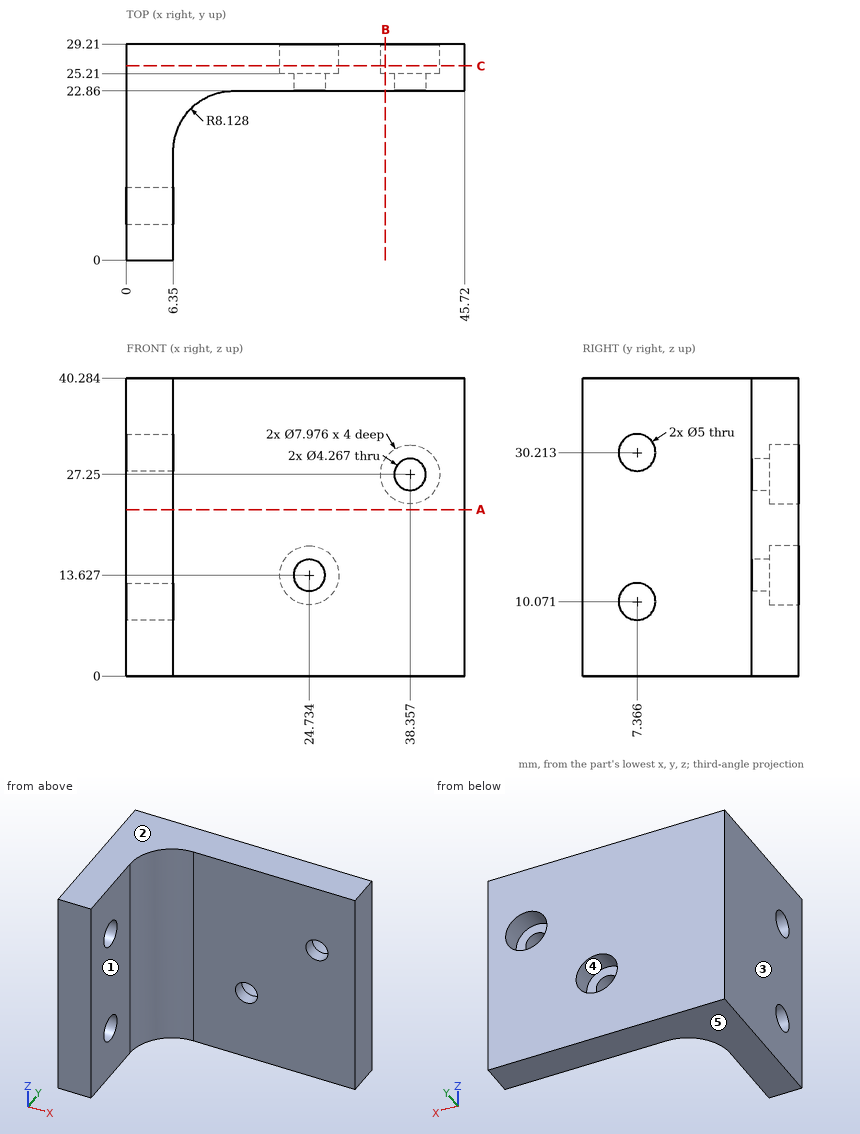
Design review of the part shown in the three views and the two pictorial views. Dimensions are in mm from the part's minimum x, y and z. A direction names the side the tool comes from. Give positions to 0.01 mm unless a question says otherwise; leave off trailing zeros. Write each loop counter-clockwise with the first axis right and the second up, starting at its lowest first coordinate (ties: lowest second). Pieces come first, ordered by that corner, then holes. Notation, with made-up numbers: M 16,15.5 L 32,15.5 A15 cw 32,42.5 Z; hole C -17,-29.75 d3. An arc over 180 degrees is marked long. One line per item, written item: value.
1) For line 1 (Y direction, x = 28, z = 33); line 2 (X direction, y = 11, z = 23.5); line 3 (Z direction, x = 5.5, y = 9.5) (1 decimal), list the stretches that pass through material, from the lowest coordinate up. Write a range as from..to.
Results are:
line 1: y = 22.86..29.21
line 2: x = 0..6.35
line 3: z = 0..8.8, 11.4..28.9, 31.5..40.3
2) Take a section at C-C, the plane y = 26.25. Count the separate pieces of the cut face and the enclosed holes in it, then the cut area to 3 significant figures.
Results are:
separate pieces: 1
enclosed holes: 2
area: 1,740 mm²
3) Take a section at B-B, the plane x = 35. Write out the cut boundary in (y, z) (1 decimal).
Results are:
outline: M 22.9,0 L 29.2,0 L 29.2,25.1 L 25.2,25.1 L 25.2,29.4 L 29.2,29.4 L 29.2,40.3 L 22.9,40.3 Z
4) For the marked faces 1 and 2, list the 3-axis set-ups (+Z, -Z, +X, -X, +Y, -Y) from which the entire face can be reached by the end or side of a thin tool; tool diameter is ignored.
Results are:
face 1: +Z, -Z, +X, -Y
face 2: +Z, +X, -X, +Y, -Y
5) Take a section at A-A, the plane z = 22.5. Write out the cut boundary in (x, y), then the cut area to 3 significant figures.
Results are:
outline: M 0,0 L 6.35,0 L 6.35,14.73 A8.13 cw 14.48,22.86 L 45.72,22.86 L 45.72,29.21 L 0,29.21 Z
area: 450 mm²
6) For P1, Ø5, axis at y = 15, z = 23, coming from the +X side (1 decimal); P2, Ø9, axis at x = 24.5, z = 14.5, coming from the +Y side; P3, Ø5, axis at y = 3, z = 21, coming from the +X side; P4, Ø7, axis at x = 24.73, z = 13.63, coming from the +Y side, all flat-tipped, find the tip position at first contact; note any pin that passes through.
Results are:
P1: stops at x = 6.8
P2: stops at y = 29.21
P3: stops at x = 6.35
P4: stops at y = 25.21
7) The part is to be moulded in two halves that separate along Z. For the marked faces 3, 4 and 5, say which applies: +Z half, -Z half, draft (parallel to the pull), parting line (faces both ways), or undercut.
Results are:
face 3: draft
face 4: undercut
face 5: -Z half
